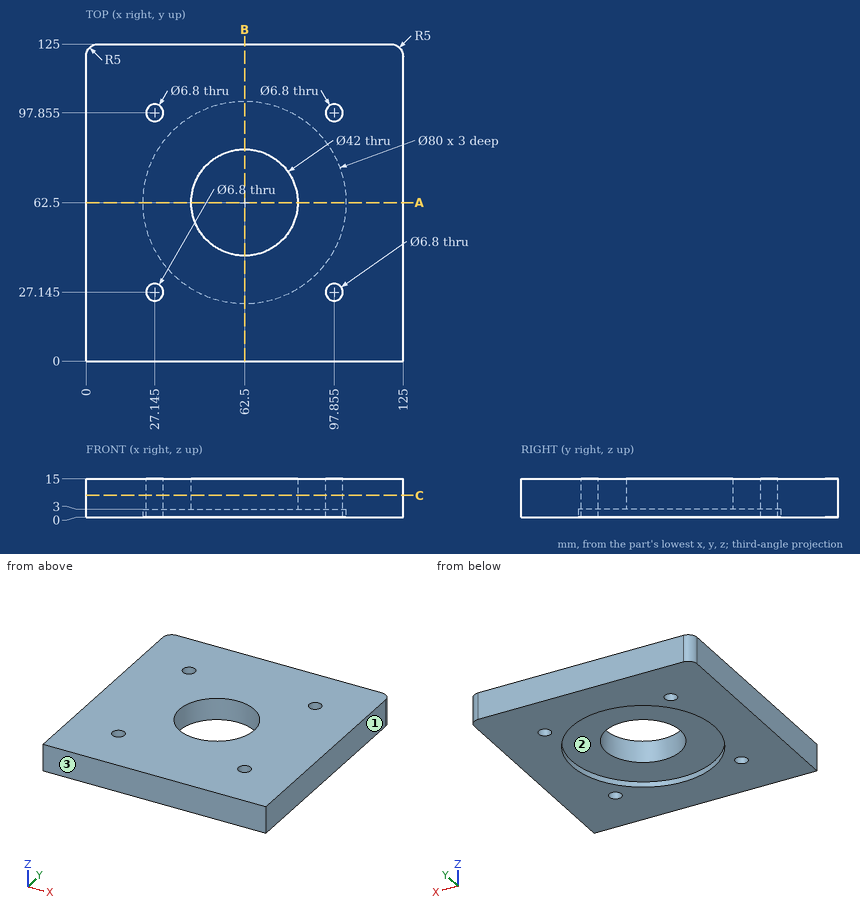
Geometry check sheet. Reference: drawing and pictorial views, mm from the part's lowest x, y, z. Coordinates: 2 decimals unless noted, no trailing zeros. Order: outer loops, then holes, each group sorted by start corner. A loop starts at its lowest first (then second) coordinate and runs counter-clockwise, first axis right, second up. Notation, with made-up numbers: M 67,73.5 L 98,73.5 A13 cw 98,81.5 Z; hole C 79,27.5 d10. An arc over 180 degrees is marked long. Return JSON: item names as keys, results as strings.
1) Release check for a two-part mould opening along Y. For the marked faces 1, 2 and 3 record: +Y half, -Y half, draft (parallel to the pull), parting line (faces both ways), or undercut.
Answer list:
{"face 1": "draft", "face 2": "undercut", "face 3": "-Y half"}
2) Thickness scan on L1, parallel to Y at x = 62.5, z = 6.5; L2, parallel to X at y = 62, z = 9.5; L3, parallel to X at y = 29.5, z = 2.5 (1 decimal). Record the ranges inside material, lowest first. Write a range as [from, to].
Answer list:
{"L1": "[0, 41.5], [83.5, 125]", "L2": "[0, 41.51], [83.49, 125]", "L3": "[0, 24.7], [29.6, 39.9], [85.1, 95.4], [100.3, 125]"}
3) Cross-section at A-A, the plane y = 62.5. Record the boundary of the cut face in (x, z), and give its area (3 significant figures).
Answer list:
{"outline": "M 0,0 L 22.5,0 L 22.5,3 L 41.5,3 L 41.5,15 L 0,15 Z; M 83.5,3 L 102.5,3 L 102.5,0 L 125,0 L 125,15 L 83.5,15 Z", "area": "1,130 mm2"}
4) Cross-section at C-C, the plane z = 8.5. Record the boundary of the cut face in (x, y) (1 decimal), and give its area (3 significant figures).
Answer list:
{"outline": "M 0,0 L 125,0 L 125,120 A5 ccw 120,125 L 5,125 A5 ccw 0,120 Z; hole C 27.1,27.1 d6.8; hole C 27.1,97.9 d6.8; hole C 62.5,62.5 d42; hole C 97.9,27.1 d6.8; hole C 97.9,97.9 d6.8", "area": "14,100 mm2"}
